from build123d import *


with BuildPart() as f2:
    # F2: sweep along a path in F0
    with BuildLine(Plane.XY) as f2_path:
        Line((43.8491681264, 31.8582854615), (54.2005525611, 0))
        Line((54.2005525611, 0), (43.8491681264, -31.8582854615))
        Line((43.8491681264, -31.8582854615), (16.7488918459, -51.5477887))
        Line((16.7488918459, -51.5477887), (-16.7488918459, -51.5477887))
        Line((-16.7488918459, -51.5477887), (-43.8491681264, -31.8582854615))
        Line((-43.8491681264, -31.8582854615), (-54.2005525611, 0))
        Line((-54.2005525611, 0), (-43.8491681264, 31.8582854615))
        Line((-43.8491681264, 31.8582854615), (-16.7488918459, 51.5477887))
        Line((-16.7488918459, 51.5477887), (16.7488918459, 51.5477887))
        Line((16.7488918459, 51.5477887), (43.8491681264, 31.8582854615))
    # F1 (on Front) → F2 (sweep)
    with BuildSketch(Plane.XZ):
        Polygon((45.676918445, 13.4097485954), (49.2700497519, 0), (54.2005525611, 0), (49.9468591312, 15.875), (27.7218591312, 38.1), (15.0218591312, 38.1), (15.0218591312, 33.3375), (25.7491670404, 33.3375), align=None)
    sweep(path=f2_path.line, transition=Transition.RIGHT)


solid = f2.part
Verification items for the finished model (mm, model axes). A direction names the side the tool comes from. Give positions to 0.01 mm unless a question says otherwise; leave off trailing zeros. Order: outer loops, then holes, each group sorted by start corner. A loop starts at its lowest first (then second) coordinate and runs counter-clockwise, first axis right, second up. Notation, with made-up numbers: M 70,47 L 128,47 A21 ccw 128,86 Z; hole C 29.25,76 d9. An arc over 180 degrees is marked long. Use one line per item in the form item = value. Start each with the question number.
Q1. Scan lines: line 1 along X through (y, z) = (-26, 10.5); line 2 along Y through (x, z) = (1.5, 9.5); line 3 along X through (y, z) = (-12.5, 7). Record each from-to range of solid material in increasing order. Write a range as [from, to].
Q2. Mould release check, pull along X, two halves, no side actions. Record for faces 1 (the flat face through (-0.42, -37.57, 26.32)), 2 (the flat face through (-22.42, -30.15, 26.32)), 3 (the flat face through (13.567, -4.477, 35.752)): +X half, -X half, draft (parallel to the pull), parting line (faces both ways), or undercut.
Q3. Section check A-A (x = 2). Enter the section's corners in (y, z) (1 decimal), then the cut area to 3 significant figures.
Q4. Section check C-C (y = 36.5). Enter the section's corners in (x, z) (3 decimals), then the cut area to 3 significant figures.
Q5. Access from +Z, -Z, +X, -X, +Y, -Y to the whole of each face (thin tool, end or side, straight path). Record for faces 4 (the flat face through (26.3, 36.7, 6.7)), 5 (the flat face through (-0.405, 49.579, 7.726)), 6 (the flat face through (13.61, 4.35, 35.75)).
Q6. Go/stop test with flat-tipped pins: pin 1 Ø4 at (x, y) = (-34, 24.5) entering from +Z; pin 2 Ø12 at (y, z) = (31, 30.5) entering from +X; pin 3 Ø1 at (x, z) = (23, 21.5) entering from +Y. Record where each tip stops, or that it passes through.
Q7. Section check B-B (z = 8.5). Enter the section's corners in (x, y).
Q8. Section check D-D (y = -6). Enter the section's corners in (x, z) (1 decimal).
Evaluation:
q1.line_1 = [-42.94, -38.01], [38.01, 42.94]
q1.line_2 = [-49.13, -44.44], [44.44, 49.13]
q1.line_3 = [-48.26, -43.33], [43.33, 48.26]
q2.face_1 = draft
q2.face_2 = -X half
q2.face_3 = undercut
q3.outline = M -51.5,0 L -46.9,0 L -43.4,13.4 L -24.5,33.3 L -14.3,33.3 L -14.3,38.1 L -26.4,38.1 L -47.5,15.9 Z; M 14.3,33.3 L 24.5,33.3 L 43.4,13.4 L 46.9,0 L 51.5,0 L 47.5,15.9 L 26.4,38.1 L 14.3,38.1 Z
q3.area = 513 mm2
q4.outline = M -37.46,0 L -29.483,0 L -23.669,13.41 L -11.86,20.708 L 11.86,20.708 L 23.669,13.41 L 29.483,0 L 37.46,0 L 30.578,15.875 L 11.86,27.443 L -11.86,27.443 L -30.578,15.875 Z
q4.area = 599 mm2
q5.face_4 = -Z
q5.face_5 = +Z, +X, -X, +Y
q5.face_6 = +Z, -Z
q6.pin_1 = 25.91
q6.pin_2 = 27.23
q6.pin_3 = 36.08
q7.outline = M -51.92,0 L -42.01,-30.52 L -16.05,-49.38 L 16.05,-49.38 L 42.01,-30.52 L 51.92,0 L 42.01,30.52 L 16.05,49.38 L -16.05,49.38 L -42.01,30.52 Z; hole M -46.99,0 L -38.02,-27.62 L -14.52,-44.69 L 14.52,-44.69 L 38.02,-27.62 L 46.99,0 L 38.02,27.62 L 14.52,44.69 L -14.52,44.69 L -38.02,27.62 Z
q8.outline = M -52.3,0 L -47.3,0 L -43.7,13.4 L -23.8,33.3 L -13.1,33.3 L -13.1,38.1 L -25.8,38.1 L -48,15.9 Z; M 13.1,33.3 L 23.8,33.3 L 43.7,13.4 L 47.3,0 L 52.3,0 L 48,15.9 L 25.8,38.1 L 13.1,38.1 Z
